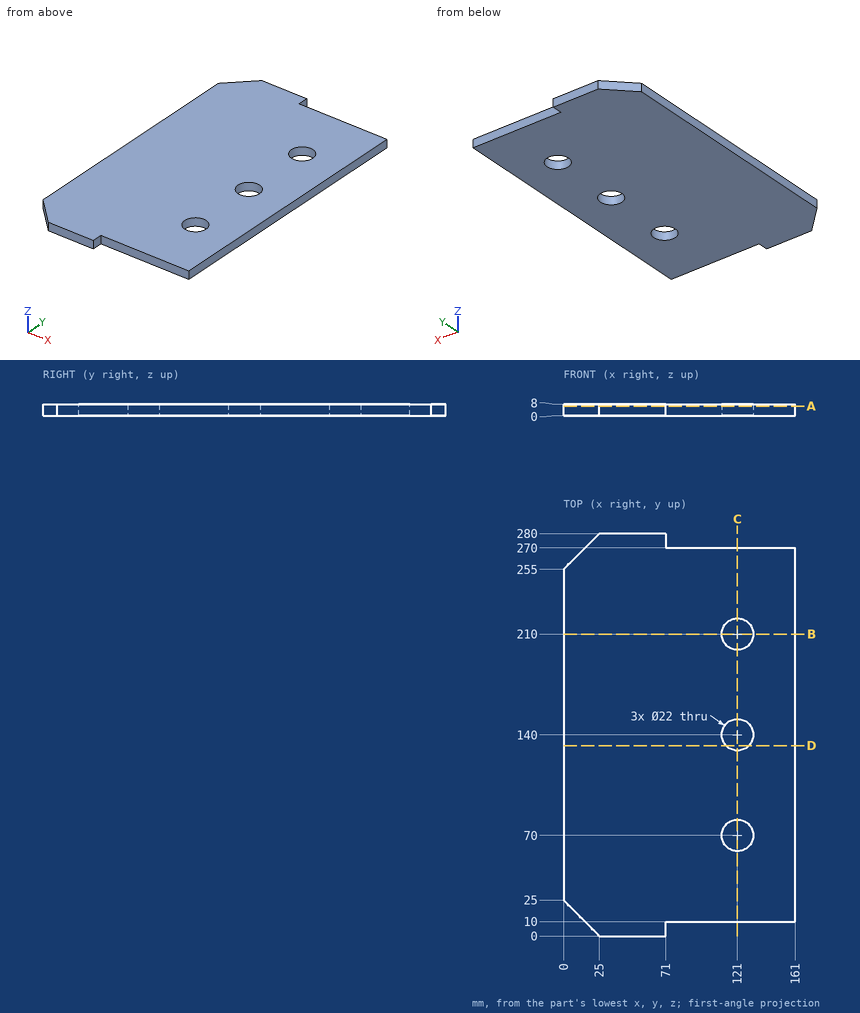
Geometry check sheet. Reference: drawing and pictorial views, mm from the part's lowest x, y, z. Give positions to 0.01 mm unless a question says otherwise; leave off trailing zeros. Order: outer loops, then holes, each group sorted by start corner. A loop starts at its lowest first (then second) coordinate and runs counter-clockwise, first axis right, second up. Notation, with made-up numbers: (-35, 70) -> (-1, 70) arc R31 ccw to (-1, 104) -> close; hole circle Ø9 at (75.5, 26). An arc over 180 degrees is marked (long way). Write each question's results on one line, items separated by ' | '. Start each with the question number.
(1) Gauge pin test, flat ends, axial feed: P1, Ø4, axis at x = 135, z = 3.5, coming from the +Y side; P2, Ø4, axis at x = 88, y = 83.5, coming from the -Z side; P3, Ø20, axis at x = 121, y = 140, coming from the +Z side. Record the tip position at first contact, or that the pin passes through.
(2) Sectioned sample at A-A (z = 6.5). Enter the section's corners in (x, y), plus the area to 3 significant figures.
(3) Scan lines: line 1 (Y direction, x = 121, z = 5.25); line 2 (X direction, y = 70, z = 2.5); line 3 (Y direction, x = 130, z = 6.5). Record each from-to range of solid material in increasing order.
(4) Sectioned sample at B-B (y = 210). Enter the section's corners in (x, z).
(5) Sectioned sample at C-C (x = 121). Enter the section's corners in (y, z), plus the area to 3 significant figures.
(6) Sectioned sample at D-D (y = 132.5). Enter the section's corners in (x, z).
Answer below:
1) P1: y = 270 | P2: z = 0 | P3: through
2) outline: (0, 25) -> (25, 0) -> (71, 0) -> (71, 10) -> (161, 10) -> (161, 270) -> (71, 270) -> (71, 280) -> (25, 280) -> (0, 255) -> close; hole circle Ø22 at (121, 70); hole circle Ø22 at (121, 140); hole circle Ø22 at (121, 210) | area: 41,500 mm2
3) line 1: 10 to 59, 81 to 129, 151 to 199, 221 to 270 | line 2: 0 to 110, 132 to 161 | line 3: 10 to 63.68, 76.32 to 133.68, 146.32 to 203.68, 216.32 to 270
4) outline: (0, 0) -> (110, 0) -> (110, 8) -> (0, 8) -> close; (132, 0) -> (161, 0) -> (161, 8) -> (132, 8) -> close
5) outline: (10, 0) -> (59, 0) -> (59, 8) -> (10, 8) -> close; (81, 0) -> (129, 0) -> (129, 8) -> (81, 8) -> close; (151, 0) -> (199, 0) -> (199, 8) -> (151, 8) -> close; (221, 0) -> (270, 0) -> (270, 8) -> (221, 8) -> close | area: 1,550 mm2
6) outline: (0, 0) -> (112.95, 0) -> (112.95, 8) -> (0, 8) -> close; (129.05, 0) -> (161, 0) -> (161, 8) -> (129.05, 8) -> close
